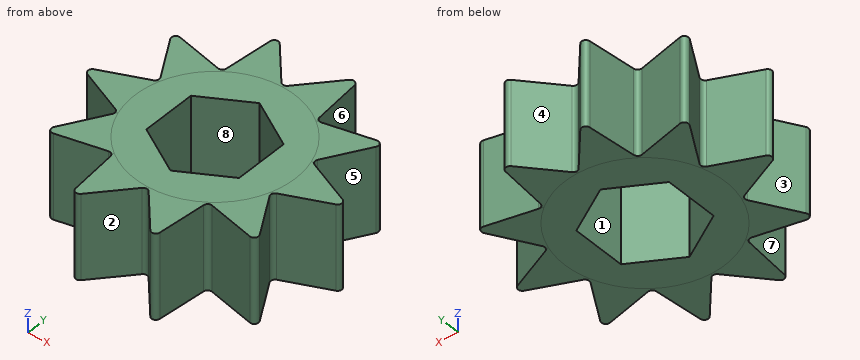
Autodesk Inventor part; units mm, degrees
ref_plane "YZ Plane" through (0, 0, 0) normal (1, 0, 0) x (0, 1, 0)
ref_plane "XZ Plane" through (0, 0, 0) normal (0, 1, 0) x (-1, 0, 0)
ref_plane "XY Plane" through (0, 0, 0) normal (0, 0, 1) x (1, 0, 0)
sketch "Sketch1" plane through (0, 0, 0) normal (0, 0, 1) x (1, 0, 0)
  circle A0 centre (0, 0) radius 2.3812 construction
  circle A1 centre (0, 0) radius 3.9687 construction
  circle A2 centre (0, 0) radius 2.3812
  circle A3 centre (0, 0) radius 2.3812
  circle A4 centre (0, 0) radius 2.3812
  circle A5 centre (0, 0) radius 2.3812
  circle A6 centre (0, 0) radius 2.3812
  circle A7 centre (0, 0) radius 2.3812
  circle A8 centre (0, 0) radius 2.3812
  circle A9 centre (0, 0) radius 2.3812
  circle A10 centre (0, 0) radius 2.3812
  line L0 (-1.3997, 1.9265) -> (-1.2264, 3.7745)
  line L1 (-1.2264, 3.7745) -> (0, 2.3812)
  line L2 (1.3997, 1.9265) -> (3.2108, 2.3328)
  line L3 (3.2108, 2.3328) -> (2.2647, 0.7358)
  line L4 (3.9687, 0) -> (2.2647, 0.7358)
  line L5 (3.9687, 0) -> (2.2647, -0.7358)
  line L6 (3.2108, -2.3328) -> (2.2647, -0.7358)
  line L7 (1.3997, -1.9265) -> (3.2108, -2.3328)
  line L8 (1.3997, -1.9265) -> (1.2264, -3.7745)
  line L9 (1.2264, -3.7745) -> (0, -2.3812)
  line L10 (-1.2264, -3.7745) -> (0, -2.3812)
  line L11 (-1.3997, -1.9265) -> (-1.2264, -3.7745)
  line L12 (-1.3997, -1.9265) -> (-3.2108, -2.3328)
  line L13 (-3.2108, -2.3328) -> (-2.2647, -0.7358)
  line L14 (-2.2647, -0.7358) -> (-3.9687, 0)
  line L15 (-3.9687, 0) -> (-2.2647, 0.7358)
  line L16 (-3.2108, 2.3328) -> (-2.2647, 0.7358)
  line L17 (-3.2108, 2.3328) -> (-1.3997, 1.9265)
  line L18 (0, 2.3812) -> (1.2264, 3.7745)
  line L19 (1.2264, 3.7745) -> (1.3997, 1.9265)
  dimension "d0" = 4.7625
  dimension "d1" = 7.9375
  dimension "d4" = 360
  dimension "d6" = 82.712
extrude "Extrusion1" add sketch "Sketch1" along normal blind 2.54
sketch "Sketch2" plane through (0, 0, 2.54) normal (0, 0, 1) x (1, 0, 0)
  line L0 (0, 1.5926) -> (1.3792, 0.7963)
  line L1 (1.3792, 0.7963) -> (1.3792, -0.7963)
  line L2 (1.3792, -0.7963) -> (0, -1.5926)
  line L3 (0, -1.5926) -> (-1.3792, -0.7963)
  line L4 (-1.3792, -0.7963) -> (-1.3792, 0.7963)
  line L5 (-1.3792, 0.7963) -> (0, 1.5926)
  point P0 (0, 0)
  point P1 (0, 0)
  dimension "d9" = 3.1852
  dimension "d10" = 1.3792
extrude "Extrusion2" cut sketch "Sketch2" against normal through all
fillet "Fillet1" radius 0.127 20 edges at (-3.2108, -2.3328, 1.27) (-3.9687, 0, 1.27) (-3.2108, 2.3328, 1.27) (-1.2264, 3.7745, 1.27) (1.2264, 3.7745, 1.27) (3.2108, 2.3328, 1.27) (3.9687, 0, 1.27) (3.2108, -2.3328, 1.27) (1.2264, -3.7745, 1.27) (-1.2264, -3.7745, 1.27) (0, -2.3812, 1.27) (1.3997, -1.9265, 1.27) (2.2647, 0.7358, 1.27) (2.2647, -0.7358, 1.27) (1.3997, 1.9265, 1.27) (0, 2.3812, 1.27) (-1.3997, 1.9265, 1.27) (-2.2647, 0.7358, 1.27) (-2.2647, -0.7358, 1.27) (-1.3997, -1.9265, 1.27)
properties part number "000113"
Here's how the part is built. I have some questions about the finished solid (model axes, mm). Face numbers are marked on the shaded views. A direction names the side the tool comes from. Round coordinates to 2 decimals unless told otherwise and drop trailing zeros. Order: outer loops, then holes, each group sorted by start corner. A loop starts at its lowest first (then second) coordinate and runs counter-clockwise, first axis right, second up. Notation, with made-up numbers: (82, 88.5) -> (135, 88.5) arc R13 ccw to (135, 94.5) -> close; hole circle Ø1 at (-25.75, 20). An arc over 180 degrees is marked (long way). Use CSV: the item, a comma, the result in double quotes.
1. I need wall thicknesses on line 1 along Y through (x, z) = (2.5, 2.05); line 2 along Y through (x, z) = (-2.75, 1.45); line 3 along X through (y, z) = (-3, 2.2). Which ranges of each line are inside material? Lowest first, please.
Recorded:
line 1,"y = -2.17 to -1.13, -0.63 to 0.63, 1.13 to 2.17"
line 2,"y = -2.23 to -1.55, -0.53 to 0.53, 1.55 to 2.23"
line 3,"x = -1.3 to -0.54, 0.54 to 1.3"
2. I want a section at B-B on y = 0.25. List the corners of the cut face in (x, z) for me, and give its area (3 significant figures).
Recorded:
outline,"(-3.39, 0) -> (-1.38, 0) -> (-1.38, 2.54) -> (-3.39, 2.54) -> close; (1.38, 0) -> (3.39, 0) -> (3.39, 2.54) -> (1.38, 2.54) -> close"
area,"10.2 mm2"
3. I want a section at C-C on y = 1.75. List the corners of the cut face in (x, z) for me.
Recorded:
outline,"(-2.87, 0) -> (2.87, 0) -> (2.87, 2.54) -> (-2.87, 2.54) -> close"
4. Which directions (+Z, -Z, +X, -X, +Y, -Y) give clear straight access to the entire face, cutting with the end or side of a thin tool? Please do the marked faces 1, 2, 3 and 4.
Recorded:
face 1,"+Z, -Z"
face 2,"+Z, -Z, -Y"
face 3,"+Z, -Z, -X"
face 4,"+Z, -Z, +Y"
5. I want a section at A-A on x = -0.75. List the corners of the cut face in (y, z) for me, and give its area (3 significant figures).
Recorded:
outline,"(-3.23, 0) -> (-1.16, 0) -> (-1.16, 2.54) -> (-3.23, 2.54) -> close; (1.16, 0) -> (3.23, 0) -> (3.23, 2.54) -> (1.16, 2.54) -> close"
area,"10.5 mm2"
6. I want a section at D-D on x = -3.25. List the corners of the cut face in (y, z) for me.
Recorded:
outline,"(-0.31, 0) -> (0.31, 0) -> (0.31, 2.54) -> (-0.31, 2.54) -> close"
7. I'm going to push a flat-ended pin straight in: P1, Ø1, axis at y = 2.5, z = 2, coming from the +X side. Where does the tip first touch, or does it pass through?
Recorded:
P1,"stops at x = 3.08"
8. Thinking about a two-plate mould opening in Y: for the marked faces 5, 6, 7 and 8, which applies, pulls with the +Y half, pulls with the -Y half, needs draft (parallel to the pull), parting line crosses it, or undercut?
Recorded:
face 5,"undercut"
face 6,"pulls with the +Y half"
face 7,"pulls with the -Y half"
face 8,"undercut"
